Here's how the part is built. I have some questions about the finished solid (model axes, mm). Coordinates: 2 decimals unless noted, no trailing zeros. Loops run counter-clockwise (first coordinate to the right, second up) from the corner with the lowest first, then second, coordinate; pieces in that order, holes last. Notation, with made-up numbers: M 44,55.5 L 74,55.5 A13 ccw 74,78.5 Z; hole C 53.5,35 d10. An arc over 180 degrees is marked long. Use CSV: the item, a comma, the result in double quotes. Start each with the question number.
Q1. If we section it at B-B (z = 2.3): State how many separate pieces and enclosed holes the cut face has, and give its area (3 significant figures).
Q2. Please list where these lines run through material, in increasing order: probe 1 along Y at (x, z) = (6.35, 1.35); probe 2 along X at (y, z) = (8.25, 0.55); probe 3 along X at (y, z) = (3.75, 0.75). Write a range as [from, to].
Q3. If we section it at A-A (y = 6.35): Please give me the cut outline in (x, z) (1 decimal), and give its area (3 significant figures).
Q4. If we section it at C-C (x = 171.45): Please give me the cut outline in (y, z) (1 decimal).
Q5. For pin 1 Ø7.5 at (x, y) = (171.45, 6.35) entering from +Z, with a flat end and sliding along its axis, tell me the tip position at first contact or that it passes through.
from build123d import *

# Parameters (mm, degrees)
SKETCH1_W          = 177.8
SKETCH1_H          = 12.7
SKETCH1_R          = 4.7625
BASE_EXTRUDE_DEPTH = 3.175
CHAMFER1_SIZE      = 3.175


with BuildPart() as part:
    # Sketch1 → Base-Extrude (new body)
    with BuildSketch(Plane.XY):
        with Locations((88.9, 6.35)):
            Rectangle(SKETCH1_W, SKETCH1_H)
        with Locations((6.35, 6.35)):
            Circle(SKETCH1_R, mode=Mode.SUBTRACT)
        with Locations(Location((171.45, 6.35, 0), (0, 0, 180))):
            Circle(SKETCH1_R, mode=Mode.SUBTRACT)
    extrude(amount=BASE_EXTRUDE_DEPTH)

    # Chamfer1
    chamfer1_edges = [part.edges().sort_by_distance(p)[0] for p in [
        (0, 12.7, 1.5875),
        (177.8, 12.7, 1.5875),
        (177.8, 0, 1.5875),
        (0, 0, 1.5875),
    ]]
    chamfer(chamfer1_edges, length=CHAMFER1_SIZE)


solid = part.part
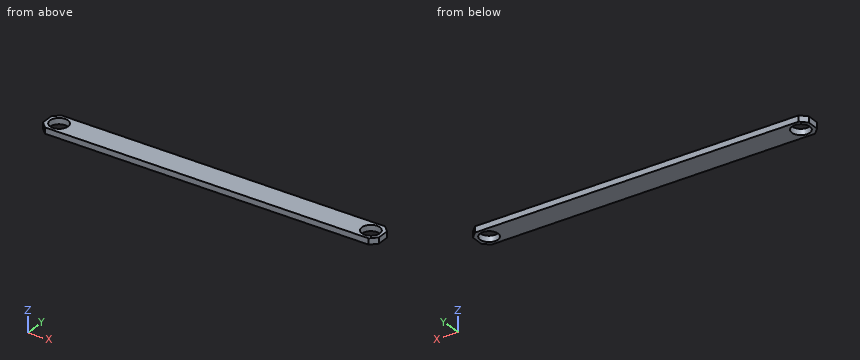
Results below:
1,separate pieces,"1"
1,enclosed holes,"2"
1,area,"2,100 mm^2"
2,probe 1,"[0, 1.59], [11.11, 12.7]"
2,probe 2,"[0, 1.98], [10.72, 167.08], [175.82, 177.8]"
2,probe 3,"[0, 2.36], [10.34, 167.46], [175.44, 177.8]"
3,outline,"M 0,0 L 1.6,0 L 1.6,3.2 L 0,3.2 Z; M 11.1,0 L 166.7,0 L 166.7,3.2 L 11.1,3.2 Z; M 176.2,0 L 177.8,0 L 177.8,3.2 L 176.2,3.2 Z"
3,area,"504 mm^2"
4,outline,"M 0,0 L 1.6,0 L 1.6,3.2 L 0,3.2 Z; M 11.1,0 L 12.7,0 L 12.7,3.2 L 11.1,3.2 Z"
5,pin 1,"through"
